```python
from build123d import *

# Parameters (mm, degrees)
F1_DEPTH = 3
F2_R     = 1


with BuildPart() as f1:
    # F0 (on Top) → F1 (new body)
    with BuildSketch(Plane.XY):
        Polygon((35, -5), (50, -5), (50, 5), (35.15, 5), (37.75, 1), (27.45, 1), (30.05, 5), (-30.05, 5), (-27.45, 1), (-37.75, 1), (-35.15, 5), (-50, 5), (-50, -5), (-35, -5), (-30.2, -5), (30.2, -5), align=None)
        Polygon((-28.05, -9), (-30.2, -5), (-35, -5), (-37.15, -9), align=None)
        Polygon((37.15, -9), (35, -5), (30.2, -5), (28.05, -9), align=None)
    extrude(amount=F1_DEPTH)

    # F2
    f2_edges = [f1.edges().sort_by_distance(p)[0] for p in [
        (-28.05, -9, 1.5),
        (-37.15, -9, 1.5),
        (37.15, -9, 1.5),
        (28.05, -9, 1.5),
        (30.05, 5, 1.5),
        (-35.15, 5, 1.5),
        (-30.05, 5, 1.5),
        (35.15, 5, 1.5),
    ]]
    fillet(f2_edges, radius=F2_R)


solid = f1.part
```
Check sheet for the modelled part. Datum: model origin and axes. Units: mm. A direction names the side the tool comes from. Round coordinates to 2 decimals unless told otherwise and drop trailing zeros. Order: outer loops, then holes, each group sorted by start corner. A loop starts at its lowest first (then second) coordinate and runs counter-clockwise, first axis right, second up. Notation, with made-up numbers: M 28.5,70.25 L 42.5,70.25 A12 cw 42.5,74.25 Z; hole C 21.25,84.5 d11. An arc over 180 degrees is marked long. Answer in a Markdown table with one row per item.
(1) Section check C-C on y = -6.5. Record the boundary of the cut face in (x, z).
Findings:
| item | result |
|---|---|
| outline | M -35.81,0 L -29.39,0 L -29.39,3 L -35.81,3 Z; M 29.39,0 L 35.81,0 L 35.81,3 L 29.39,3 Z |
(2) Material ranges on line 1 along X through (y, z) = (4, 1.6); line 2 along X through (y, z) = (1.25, 1.7); line 3 along Y through (x, z) = (40, 1.4), recorded low to high. Write a range as from..to.
Findings:
| item | result |
|---|---|
| line 1 | x = -50..-35.99, -29.21..29.21, 35.99..50 |
| line 2 | x = -50..-37.59, -27.61..27.61, 37.59..50 |
| line 3 | y = -5..5 |
(3) Section check A-A on y = 2.5. Record the boundary of the cut face in (x, z) (3 decimals).
Findings:
| item | result |
|---|---|
| outline | M -50,0 L -36.775,0 L -36.775,3 L -50,3 Z; M -28.425,0 L 28.425,0 L 28.425,3 L -28.425,3 Z; M 36.775,0 L 50,0 L 50,3 L 36.775,3 Z |
(4) Draft check along X on faces 3 (the flat face through (-33, -9, 1)), 4 (the flat face through (-50, 0, 1)), 5 (the cylindrical face through (29.093, 4.464, 1.521)), 6 (the flat face through (0, -5, 1)). Enter one of: +X half, -X half, draft (parallel to the pull), parting line (faces both ways), or undercut.
Findings:
| item | result |
|---|---|
| face 3 | draft |
| face 4 | -X half |
| face 5 | undercut |
| face 6 | undercut |
(5) Section check B-B on z = 2.35. Record the boundary of the cut face in (x, y).
Findings:
| item | result |
|---|---|
| outline | M -50,-5 L -35,-5 L -36.36,-7.53 A1 ccw -35.48,-9 L -29.72,-9 A1 ccw -28.84,-7.53 L -30.2,-5 L 30.2,-5 L 28.84,-7.53 A1 ccw 29.72,-9 L 35.48,-9 A1 ccw 36.36,-7.53 L 35,-5 L 50,-5 L 50,5 L 36.99,5 A1 ccw 36.15,3.46 L 37.75,1 L 27.45,1 L 29.05,3.46 A1 ccw 28.21,5 L -28.21,5 A1 ccw -29.05,3.46 L -27.45,1 L -37.75,1 L -36.15,3.46 A1 ccw -36.99,5 L -50,5 Z |
(6) Section check D-D on x = -23. Record the boundary of the cut face in (y, z), plus the area to 3 significant figures.
Findings:
| item | result |
|---|---|
| outline | M -5,0 L 5,0 L 5,3 L -5,3 Z |
| area | 30.0 mm^2 |
(7) Set-up check for faces 1 (the flat face through (33, 1, 1)), 2 (the flat face through (0, 5, 1)): record each of +Z, -Z, +X, -X, +Y, -Y from which the full face is reachable in a straight line by a thin tool's end or side.
Findings:
| item | result |
|---|---|
| face 1 | +Z, -Z |
| face 2 | +Z, -Z, +X, -X, +Y |
(8) Gauge pin test, flat ends, axial feed: pin 1 (1.5 mm diameter, centred on x = 40.5, z = 2, fed in from -Y); pin 2 (2 mm diameter, centred on x = 5.5, y = -1, fed in from -Z). Record the tip position at first contact, or that the pin passes through.
Findings:
| item | result |
|---|---|
| pin 1 | stops at y = -5 |
| pin 2 | stops at z = 0 |
